Here's how the part is built. I have some questions about the finished solid (model axes, mm). A direction names the side the tool comes from. Give positions to 0.01 mm unless a question says otherwise; leave off trailing zeros. Loops run counter-clockwise (first coordinate to the right, second up) from the corner with the lowest first, then second, coordinate; pieces in that order, holes last. Notation, with made-up numbers: (56.25, 86.5) - (60.25, 86.5) arc R26 cw to (60.25, 115.5) - close; hole circle Ø2 at (-24.75, 48.5). An arc over 180 degrees is marked (long way). Use one line per item in the form item = value.
Autodesk Inventor part; units mm, degrees
ref_plane "YZ Plane" through (0, 0, 0) normal (1, 0, 0) x (0, 1, 0)
ref_plane "XZ Plane" through (0, 0, 0) normal (0, 1, 0) x (-1, 0, 0)
ref_plane "XY Plane" through (0, 0, 0) normal (0, 0, 1) x (1, 0, 0)
sketch "Sketch1" plane through (0, 0, 0) normal (0, 1, 0) x (-1, 0, 0)
  line L0 (-4, 0) -> (2, 0)
  line L1 (2, 3.4641) -> (2, -3.4641)
  arc A0 (2, 3.4641) -> (2, -3.4641) centre (0.004, 0) ccw
  point P0 (0, 0)
  dimension "d1" = 6
extrude "Extrusion1" add sketch "Sketch1" along normal blind 65
sketch "Sketch2" plane through (0, 65, 0) normal (0, 1, 0) x (1, 0, 0)
  line L0 (-2, -3.4641) -> (-2, 3.4641)
  line L1 (-2, 3.4641) -> (-2, -3.4641)
  arc A0 (-2, 3.4641) -> (-2, -3.4641) centre (0, 0) ccw
extrude "Extrusion2" add sketch "Sketch2" against normal blind 8.5
sketch "Sketch3" plane through (0, 0, 0) normal (0, -1, 0) x (1, 0, 0)
  line L0 (-2, -3.4641) -> (-2, 3.4641)
  arc A0 (-2, 3.4641) -> (-2, -3.4641) centre (0, 0) ccw
  point P0 (0, 0)
extrude "Extrusion3" add sketch "Sketch3" against normal blind 8.5
sketch "Sketch4" plane through (0, 65, 0) normal (0, 1, 0) x (1, 0, 0)
  circle A0 centre (0, 0) radius 4
  dimension "d9" = 8
extrude "Extrusion4" cut sketch "Sketch4" against normal blind 8.5
sketch "Sketch5" plane through (0, 56.5, 0) normal (0, 1, 0) x (1, 0, 0)
  circle A0 centre (0, 0) radius 4
  dimension "d12" = 8
extrude "Extrusion5" add sketch "Sketch5" along normal blind 8.5
sketch "Sketch6" plane through (0, 65, 0) normal (0, 1, 0) x (1, 0, 0)
  circle A0 centre (0, 0) radius 3
  circle A1 centre (0, 0) radius 4
  dimension "d15" = 6
  dimension "d16" = 8
extrude "Extrusion6" cut sketch "Sketch6" against normal blind 6
thread "Thread1"
chamfer "Chamfer1" distance 0.5 angle 45 1 edges at (-3, 65, 0)
chamfer "Chamfer2" distance 0.5 angle 45 1 edges at (-4, 59, 0)
sketch "Sketch7" plane through (0, 0, 0) normal (0, -1, 0) x (1, 0, 0)
  circle A0 centre (0, 0) radius 4
  dimension "d27" = 8
extrude "Extrusion7" cut sketch "Sketch7" against normal blind 4
sketch "Sketch8" plane through (0, 4, 0) normal (0, -1, 0) x (1, 0, 0)
  circle A0 centre (0, 0) radius 4
  dimension "d30" = 8
extrude "Extrusion8" add sketch "Sketch8" along normal blind 4
chamfer "Chamfer3" distance 0.5 angle 45 1 edges at (-4, 0, 0)
properties part number "hridel_senzor"
(1) For P1, Ø1.5, axis at y = 18, z = -2, coming from the +X side; P2, Ø3, axis at y = 20, z = -3, coming from the -X side; P3, Ø2, axis at y = 13, z = -1.5, coming from the +X side, each with a flat end and sliding along its axis, tell me the tip position at first contact or that it passes through.
Geometry says:
P1 = 3.79
P2 = -2
P3 = 3.96
(2) If I drill on probe 1 along Y at (x, z) = (-3.25, -0.25); probe 2 along Y at (x, z) = (-2.5, -0.25); probe 3 along Y at (x, z) = (1.25, -3.25), over which ranges is the centre line in solid material (lowest first)?
Geometry says:
probe_1 = 0 to 8.5, 56.5 to 59
probe_2 = 0 to 8.5, 56.5 to 64.99
probe_3 = 0 to 59
(3) If we section it at D-D (y = 60): List the corners of the cut face in (x, z) for me.
Geometry says:
outline = circle Ø6 at (0, 0)
(4) For faces 4 (the flat face through (0, 65, 0)), 5 (the flat face through (-3, 56.5, 0)), which set-ups out of +Z, -Z, +X, -X, +Y, -Y let a thin tool reach every point of the face, with its end or its side?
Geometry says:
face_4 = +Z, -Z, +X, -X, +Y
face_5 = +Z, -Z, -X
(5) Thinking about a two-plate mould opening in Y: for faces 1 (the flat face through (-3, 8.5, 0)), 2 (the cylindrical face through (-3, 62, 0)), 3 (the flat face through (3, 59, -1)), which applies, pulls with the +Y half, pulls with the -Y half, needs draft (parallel to the pull), parting line crosses it, or undercut?
Geometry says:
face_1 = undercut
face_2 = needs draft
face_3 = pulls with the +Y half
(6) If we section it at C-C (y = 28): List the corners of the cut face in (x, z) for me, plus the area to 3 significant figures.
Geometry says:
outline = (-2, -3.46) arc R4 ccw (long way) to (-2, 3.46) - close
area = 40.4 mm²
